from build123d import *

# Parameters (mm, degrees)
ESBO_O1_R                = 3.05
RESSALTO_EXTRUS_O1_DEPTH = 4
FILETE1_R                = 3


with BuildPart() as part:
    # Esboço1 → Ressalto-extrusão1 (new body)
    with BuildSketch(Plane.XY):
        Polygon((0, 38.263883749), (-35, 18.056624327), (-35, 12), (-25, 12), (-25, 6), (-35, 6), (-35, 0), (0, 0), (0, 6), (-10, 6), (-10, 12), (0, 12), align=None)
        with Locations((-13.767949192, 20.5)):
            Circle(ESBO_O1_R, mode=Mode.SUBTRACT)
    extrude(amount=RESSALTO_EXTRUS_O1_DEPTH)

    # Filete1
    filete1_edges = [part.edges().sort_by_distance(p)[0] for p in [
        (-35, 18.056624327, 2),
        (0, 38.263883749, 2),
    ]]
    fillet(filete1_edges, radius=FILETE1_R)


solid = part.part
The listing builds one solid part. Answer for the finished solid, in the listing's coordinates (mm). A direction names the side the tool comes from. Coordinates: 2 decimals unless noted, no trailing zeros. Loops run counter-clockwise (first coordinate to the right, second up) from the corner with the lowest first, then second, coordinate; pieces in that order, holes last. Notation, with made-up numbers: (7, 24) -> (25, 24) arc R36 cw to (25, 63) -> close; hole circle Ø5 at (24.25, 80). An arc over 180 degrees is marked (long way). Answer in a Markdown table with one row per item. Add a question column.
1. Flat-ended cylindrical pins translate along their axes: P1, Ø1.2, axis at x = -29, z = 1.5, coming from the +Y side; P2, Ø2, axis at y = 8, z = 1.5, coming from the +X side. Find the tip coordinate at first contact, or state that the pin passes through.
2. Determine the mould class of faces 4 (the cylindrical face through (-1.54, 35.69, 2.03)), 5 (the flat face through (-35, 14, 2)), 6 (the flat face through (-5, 6, 2)) for opening direction Y: +Y half, -Y half, draft (parallel to the pull), parting line (faces both ways), or undercut.
3. Consider line 1 (Y direction, x = -1.5, z = 3.7); line 2 (X direction, y = 11, z = 2.85); line 3 (Y direction, x = -32, z = 2.75). Determine where each line is inside the solid, lowest interval first. Write a range as [from, to].
4. The part is cut by section B-B, the plane z = 3.3. Write down the section's boundary in (x, y), then the cut area to 3 significant figures.
5. The part is cut by section C-C, the plane x = -11.5. Write down the section's boundary in (y, z).
6. For faces 1 (the flat face through (-10, 9, 2)), 2 (the flat face through (-25, 9, 2)), 3 (the flat face through (0, 22, 2)), determine the directions among +Z, -Z, +X, -X, +Y, -Y from which every point of the face is accessible in a straight line to the end or side of a thin tool.
7. The part is cut by section A-A, the plane y = 20.5. Write down the section's boundary in (x, z), then the cut area to 3 significant figures.
8. The part is cut by section D-D, the plane y = 9.5. Write down the section's boundary in (x, z), then the cut area to 3 significant figures.
Answer below:
| question | item | result |
|---|---|---|
| 1 | P1 | y = 21.87 |
| 1 | P2 | x = -10 |
| 2 | face 4 | +Y half |
| 2 | face 5 | draft |
| 2 | face 6 | undercut |
| 3 | line 1 | [0, 6], [12, 35.67] |
| 3 | line 2 | [-25, -10] |
| 3 | line 3 | [0, 6], [12, 19.79] |
| 4 | outline | (-35, 0) -> (0, 0) -> (0, 6) -> (-10, 6) -> (-10, 12) -> (0, 12) -> (0, 33.07) arc R3 ccw to (-4.5, 35.67) -> (-33.5, 18.92) arc R3 ccw to (-35, 16.32) -> (-35, 12) -> (-25, 12) -> (-25, 6) -> (-35, 6) -> close; hole circle Ø6.1 at (-13.77, 20.5) |
| 4 | area | 830 mm2 |
| 5 | outline | (0, 0) -> (18.46, 0) -> (18.46, 4) -> (0, 4) -> close; (22.54, 0) -> (31.62, 0) -> (31.62, 4) -> (22.54, 4) -> close |
| 6 | face 1 | +Z, -Z, +X |
| 6 | face 2 | +Z, -Z, -X |
| 6 | face 3 | +Z, -Z, +X, +Y, -Y |
| 7 | outline | (-30.77, 0) -> (-16.82, 0) -> (-16.82, 4) -> (-30.77, 4) -> close; (-10.72, 0) -> (0, 0) -> (0, 4) -> (-10.72, 4) -> close |
| 7 | area | 98.7 mm2 |
| 8 | outline | (-25, 0) -> (-10, 0) -> (-10, 4) -> (-25, 4) -> close |
| 8 | area | 60.0 mm2 |
